Model file for the job. Use its own axes, mm. Face numbers are marked on the shaded views. Round coordinates to 2 decimals unless told otherwise and drop trailing zeros. Write each loop counter-clockwise with the first axis right and the second up, starting at its lowest first coordinate (ties: lowest second). Pieces come first, ordered by that corner, then holes. Notation, with made-up numbers: (60, -36) - (71, -36) arc R23 cw to (71, -26) - close; hole circle Ø2 at (-21.5, -11.5). An arc over 180 degrees is marked (long way). One line per item, written item: value.
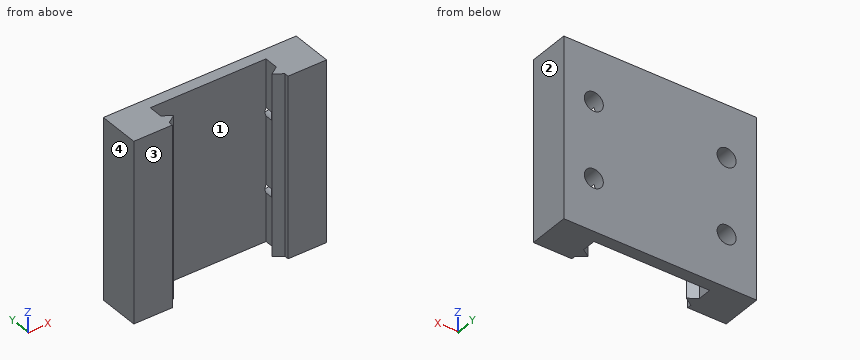
from build123d import *

# Parameters (mm, degrees)
BOSS_EXTRUDE1_DEPTH = 28.5
SKETCH2_R           = 1.5
CUT_EXTRUDE1_DEPTH  = 3


with BuildPart() as part:
    # Sketch1 → Boss-Extrude1 (new body)
    with BuildSketch(Plane.XY):
        Polygon((-9.15, -1.105576246), (-9.15, -0.419722436), (-7.770416346, 0.5), (-9.15, 1.419722436), (-9.15, 3.65), (9.15, 3.65), (9.15, 1.419722436), (7.770416346, 0.5), (9.15, -0.419722436), (9.15, -1.105576246), (15.25, -1.105576246), (15.25, 5.45289456), (-15.25, 5.45289456), (-15.25, -1.105576246), align=None)
    extrude(amount=-BOSS_EXTRUDE1_DEPTH)

    # Sketch2 → Cut-Extrude1 (cut)
    with BuildSketch(Plane(origin=(0, 5.45289456, 0), x_dir=(1, 0, 0), z_dir=(0, 1, 0))):
        with Locations((-10.5, 8.25)):
            Circle(SKETCH2_R)
        with Locations((-10.5, 20.25)):
            Circle(SKETCH2_R)
        with Locations((10.5, 20.25)):
            Circle(SKETCH2_R)
        with Locations((10.5, 8.25)):
            Circle(SKETCH2_R)
    extrude(amount=-CUT_EXTRUDE1_DEPTH, mode=Mode.SUBTRACT)


solid = part.part
1. Drop flat-ended pins along their axis: pin 1 (3 mm diameter, centred on x = 11, z = -8, fed in from +Y); pin 2 (5 mm diameter, centred on x = -2, z = -23, fed in from -Y); pin 3 (1.8 mm diameter, centred on x = 10.5, z = -8.25, fed in from +Y). Give the stop position or say it passes through.
Report:
pin 1: y = 5.45
pin 2: y = 3.65
pin 3: y = 2.45
2. Band-saw the part on C-C on y = 2. Write the cut outline in (x, z).
Report:
outline: (-15.25, -28.5) - (-9.15, -28.5) - (-9.15, 0) - (-15.25, 0) - close; (9.15, -28.5) - (15.25, -28.5) - (15.25, 0) - (9.15, 0) - close
3. Band-saw the part on A-A on z = -8.25. Write the cut outline in (x, y), plus the area to 3 significant figures.
Report:
outline: (-15.25, -1.11) - (-9.15, -1.11) - (-9.15, -0.42) - (-7.77, 0.5) - (-9.15, 1.42) - (-9.15, 2.45) - (-12, 2.45) - (-12, 5.45) - (-15.25, 5.45) - close; (-9, 3.65) - (9, 3.65) - (9, 5.45) - (-9, 5.45) - close; (7.77, 0.5) - (9.15, -0.42) - (9.15, -1.11) - (15.25, -1.11) - (15.25, 5.45) - (12, 5.45) - (12, 2.45) - (9.15, 2.45) - (9.15, 1.42) - close
area: 97.9 mm²
4. Wall check: probe 1 along Z at (x, y) = (-10.5, 3.65); probe 2 along X at (y, z) = (2.75, -2.5); probe 3 along X at (y, z) = (3.15, -20.25). Give the ranges that are in metal, low to high. Write a range as [from, to].
Report:
probe 1: [-28.5, -21.75], [-18.75, -9.75], [-6.75, 0]
probe 2: [-15.25, -9.15], [9.15, 15.25]
probe 3: [-15.25, -12], [12, 15.25]
5. Mould opens along X. For the marked faces 1, 2, 3 and 4 say: released by +X, released by -X, zero draft, split by the parting line, or undercut.
Report:
face 1: undercut
face 2: released by +X
face 3: zero draft
face 4: released by -X
6. Band-saw the part on D-D on x = 10.5. Write the cut outline in (y, z).
Report:
outline: (-1.11, -28.5) - (5.45, -28.5) - (5.45, -21.75) - (2.45, -21.75) - (2.45, -18.75) - (5.45, -18.75) - (5.45, -9.75) - (2.45, -9.75) - (2.45, -6.75) - (5.45, -6.75) - (5.45, 0) - (-1.11, 0) - close
7. Band-saw the part on B-B on y = 5. Write the cut outline in (x, z).
Report:
outline: (-15.25, -28.5) - (15.25, -28.5) - (15.25, 0) - (-15.25, 0) - close; hole circle Ø3 at (-10.5, -20.25); hole circle Ø3 at (-10.5, -8.25); hole circle Ø3 at (10.5, -20.25); hole circle Ø3 at (10.5, -8.25)
